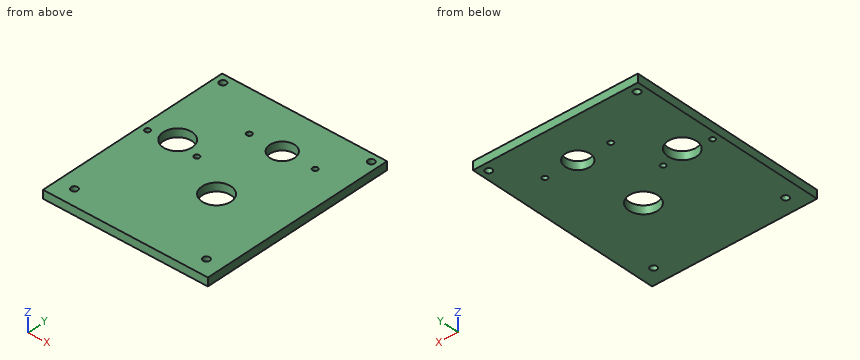
Autodesk Inventor part; units mm, degrees
ref_plane "YZ Plane" through (0, 0, 0) normal (1, 0, 0) x (0, 1, 0)
ref_plane "XZ Plane" through (0, 0, 0) normal (0, 1, 0) x (-1, 0, 0)
ref_plane "XY Plane" through (0, 0, 0) normal (0, 0, 1) x (1, 0, 0)
sketch "Sketch1" plane through (0, 0, 0) normal (0, 0, 1) x (1, 0, 0)
  circle A0 centre (0, 0) radius 9.525
  line L0 (0, 0) -> (25.4, 0) construction
  line L1 (25.4, 0) -> (-25.4, 0) construction
  line L2 (0, 0) -> (0, -55.88) construction
  line L3 (0, -55.88) -> (-51.7955, -31.7274) construction
  circle A1 centre (0, -55.88) radius 11.1125
  circle A2 centre (-51.7955, -31.7274) radius 11.1125
  line L4 (0, -55.88) -> (0, -106.68) construction
  line L5 (0, -106.68) -> (50.8, -106.68)
  line L6 (50.8, -106.68) -> (50.8, 33.02)
  line L7 (-51.7955, -31.7274) -> (-98.7855, -31.7274) construction
  line L8 (50.8, 33.02) -> (-76.2, 33.02)
  line L9 (-76.2, 33.02) -> (-76.2, -106.68)
  line L10 (-76.2, -106.68) -> (0, -106.68)
  circle A3 centre (25.4, 0) radius 2.0193
  circle A4 centre (-25.4, 0) radius 2.0193
  line L11 (-76.2, 33.02) -> (-69.85, 33.02) construction
  line L12 (-69.85, 33.02) -> (-69.85, 26.67) construction
  circle A5 centre (-69.85, 26.67) radius 2.5797
  line L13 (-12.7, 33.02) -> (-12.7, -106.68) construction
  line L14 (50.8, -36.83) -> (-76.2, -36.83) construction
  circle A6 centre (44.45, 26.67) radius 2.5797
  dimension "d0" = 19.05
  dimension "d1" = 25.4
  dimension "d2" = 50.8
  dimension "d3" = 55.88
  dimension "d4" = 57.15
  dimension "d5" = 65
  dimension "d6" = 22.225
  dimension "d7" = 22.225
  dimension "d8" = 50.8
  dimension "d9" = 50.8
  dimension "d10" = 139.7
  dimension "d11" = 46.99
  dimension "d12" = 127
  dimension "d13" = 4.0386
  dimension "d14" = 6.35
  dimension "d15" = 6.35
  dimension "d16" = 5.1594
extrude "Extrusion1" add sketch "Sketch1" along normal blind 6.35
sketch "Sketch2" plane through (0, 0, 6.35) normal (0, 0, 1) x (1, 0, 0)
  line L0 (-76.2, -106.68) -> (50.8, -106.68)
  line L1 (-76.2, -106.68) -> (50.8, -106.68)
  line L2 (50.8, -106.68) -> (50.8, -119.38)
  line L3 (50.8, -119.38) -> (-76.2, -119.38)
  line L4 (-76.2, -119.38) -> (-76.2, -106.68)
  point P0 (0, 0)
  dimension "d19" = 127
  dimension "d20" = 12.7
extrude "Extrusion2" add sketch "Sketch2" against normal blind 6.35
sketch "Sketch3" plane through (0, 0, 6.35) normal (0, 0, 1) x (1, 0, 0)
  line L0 (50.8, 33.02) -> (50.8, -119.38)
  line L1 (50.8, -119.38) -> (38.1, -119.38) construction
  line L2 (50.8, -119.38) -> (-76.2, -119.38)
  line L3 (38.1, -119.38) -> (38.1, -106.68) construction
  line L4 (-12.7, -119.38) -> (-12.7, -74.0857) construction
  circle A0 centre (38.1, -106.68) radius 2.5797
  circle A1 centre (-63.5, -106.68) radius 2.5797
  point P0 (0, 0)
  dimension "d23" = 12.7
  dimension "d24" = 12.7
  dimension "d25" = 5.1594
extrude "Extrusion3" cut sketch "Sketch3" against normal blind 6.35
sketch "Sketch4" plane through (0, 0, 6.35) normal (0, 0, 1) x (1, 0, 0)
  circle A0 centre (-51.7955, -31.7274) radius 11.1125
  circle A1 centre (-51.7955, -31.7274) radius 11.1125
  line L0 (-51.7955, -31.7274) -> (-70.8455, -31.7274) construction
  line L1 (-70.8455, -31.7274) -> (-32.7455, -31.7274) construction
  line L2 (-32.7455, -31.7274) -> (-32.7455, -36.5026) construction
  line L3 (-51.7955, -31.7274) -> (-51.7955, -49.632) construction
  circle A2 centre (-32.7455, -36.5026) radius 2.0193
  circle A3 centre (-70.8455, -36.5026) radius 2.0193
  point P0 (0, 0)
  dimension "d28" = 19.05
  dimension "d29" = 38.1
  dimension "d30" = 4.7752
  dimension "d31" = 4.0386
extrude "Extrusion4" cut sketch "Sketch4" against normal blind 6.35 contours A2 | A3
properties part number "Rack and Pinion Gearbox Plate"
Geometry: final body of the model. Coordinates: model frame, mm. Give positions to 0.01 mm unless a question says otherwise; leave off trailing zeros. Write each loop counter-clockwise with the first axis right and the second up, starting at its lowest first coordinate (ties: lowest second). Pieces come first, ordered by that corner, then holes. Notation, with made-up numbers: (65.5, -0.75) -> (123.5, -0.75) arc R23 cw to (123.5, 21.25) -> close; hole circle Ø7 at (-32, 44.25). An arc over 180 degrees is marked (long way). Answer in a Markdown table with one row per item.
(1) Section query C-C on y = 0. Return loops of the section in (x, z) (3 decimals), then the cut area to 3 significant figures.
Answers below:
| item | result |
|---|---|
| outline | (-76.2, 0) -> (-27.419, 0) -> (-27.419, 6.35) -> (-76.2, 6.35) -> close; (-23.381, 0) -> (-9.525, 0) -> (-9.525, 6.35) -> (-23.381, 6.35) -> close; (9.525, 0) -> (23.381, 0) -> (23.381, 6.35) -> (9.525, 6.35) -> close; (27.419, 0) -> (50.8, 0) -> (50.8, 6.35) -> (27.419, 6.35) -> close |
| area | 634 mm^2 |
(2) Section query D-D on y = -55.88. Return loops of the section in (x, z), then the cut area to 3 significant figures.
Answers below:
| item | result |
|---|---|
| outline | (-76.2, 0) -> (-11.11, 0) -> (-11.11, 6.35) -> (-76.2, 6.35) -> close; (11.11, 0) -> (50.8, 0) -> (50.8, 6.35) -> (11.11, 6.35) -> close |
| area | 665 mm^2 |
(3) Section query B-B on y = 26.67. Return loops of the section in (x, z), then the cut area to 3 significant figures.
Answers below:
| item | result |
|---|---|
| outline | (-76.2, 0) -> (-72.43, 0) -> (-72.43, 6.35) -> (-76.2, 6.35) -> close; (-67.27, 0) -> (41.87, 0) -> (41.87, 6.35) -> (-67.27, 6.35) -> close; (47.03, 0) -> (50.8, 0) -> (50.8, 6.35) -> (47.03, 6.35) -> close |
| area | 741 mm^2 |
(4) Pin query (flat end, axial travel): pin 1 (8.5 mm diameter, centred on x = 38.1, y = -106.68, fed in from -Z). Return the tip coordinate at first contact, or that it passes through.
Answers below:
| item | result |
|---|---|
| pin 1 | z = 0 |
(5) Ray query, line 1 along Y through (x, z) = (0, 4) (1 decimal); line 2 along X through (y, z) = (-106, 1.75); line 3 along Y through (x, z) = (-6.5, 4.25). Return the intervals inside material, ascending. Write a range as [from, to].
Answers below:
| item | result |
|---|---|
| line 1 | [-119.4, -67], [-44.8, -9.5], [9.5, 33] |
| line 2 | [-76.2, -65.99], [-61.01, 35.61], [40.59, 50.8] |
| line 3 | [-119.38, -64.89], [-46.87, -6.96], [6.96, 33.02] |
(6) Section query A-A on x = -25.4. Return loops of the section in (y, z), then the cut area to 3 significant figures.
Answers below:
| item | result |
|---|---|
| outline | (-119.38, 0) -> (-2.02, 0) -> (-2.02, 6.35) -> (-119.38, 6.35) -> close; (2.02, 0) -> (33.02, 0) -> (33.02, 6.35) -> (2.02, 6.35) -> close |
| area | 942 mm^2 |
